```python
from build123d import *

# Parameters (mm, degrees)
SKETCH1_W                   = 57.3
SKETCH1_H                   = 42
BOSS_EXTRUDE1_DEPTH         = 6.35
TAP_DRILL_FOR_M3X0_5_TAP1_D = 3.25
CUT_EXTRUDE1_DEPTH          = 37.085246293
SKETCH5_W                   = 7.65
SKETCH5_H                   = 14.65
CUT_EXTRUDE2_DEPTH          = 37.085246293
FILLET1_R                   = 5


with BuildPart() as part:
    # Sketch1 → Boss-Extrude1 (new body)
    with BuildSketch(Plane.XY):
        Rectangle(SKETCH1_W, SKETCH1_H)
    extrude(amount=BOSS_EXTRUDE1_DEPTH)

    # Tap Drill for M3x0.5 Tap1 (through all)
    with Locations(Plane.XY.offset(6.35)):
        with Locations((15.5, 15.5), (15.5, -15.5), (-15.5, 15.5), (-15.5, -15.5)):
            Hole(TAP_DRILL_FOR_M3X0_5_TAP1_D / 2)

    # Sketch4 → Cut-Extrude1 (cut, through all)
    with BuildSketch(Plane.XY.offset(6.35)):
        with BuildLine():
            ThreePointArc((11, 0), (8.93028555, 6.422616289), (3.5, 10.428326807))
            Line((3.5, 10.428326807), (-3.5, 10.428326807))
            ThreePointArc((-3.5, 10.428326807), (-6.422616289, -8.93028555), (11, 0))
        make_face()
        with BuildLine():
            Line((-3.5, 10.428326807), (3.5, 10.428326807))
            ThreePointArc((3.5, 10.428326807), (0, 11), (-3.5, 10.428326807))
        make_face()
        with BuildLine():
            ThreePointArc((-3.5, 10.428326807), (0, 11), (3.5, 10.428326807))
            Line((3.5, 10.428326807), (3.5, 21))
            Line((3.5, 21), (-3.5, 21))
            Line((-3.5, 21), (-3.5, 10.428326807))
        make_face()
    extrude(amount=-CUT_EXTRUDE1_DEPTH, mode=Mode.SUBTRACT)

    # Sketch5 → Cut-Extrude2 (cut, through all)
    with BuildSketch(Plane.XY.offset(6.35)):
        with Locations((-24.825, 13.675)):
            Rectangle(SKETCH5_W, SKETCH5_H)
        with Locations((-24.825, -13.675)):
            Rectangle(SKETCH5_W, SKETCH5_H)
    cut_extrude2 = extrude(amount=-CUT_EXTRUDE2_DEPTH, mode=Mode.SUBTRACT)

    # Mirror1: Cut-Extrude2 across plane
    add(cut_extrude2.mirror(Plane(origin=(0, 0, 0), x_dir=(0, 0, 1), z_dir=(1, 0, 0))), mode=Mode.SUBTRACT)

    # Fillet1
    fillet1_edges = [part.edges().sort_by_distance(p)[0] for p in [
        (3.5, 10.428326807, 3.175),
        (-3.5, 10.428326807, 3.175),
        (-3.5, 21, 3.175),
        (3.5, 21, 3.175),
        (-21, 21, 3.175),
        (-21, -21, 3.175),
        (21, 21, 3.175),
        (21, -21, 3.175),
    ]]
    fillet(fillet1_edges, radius=FILLET1_R)


solid = part.part
```
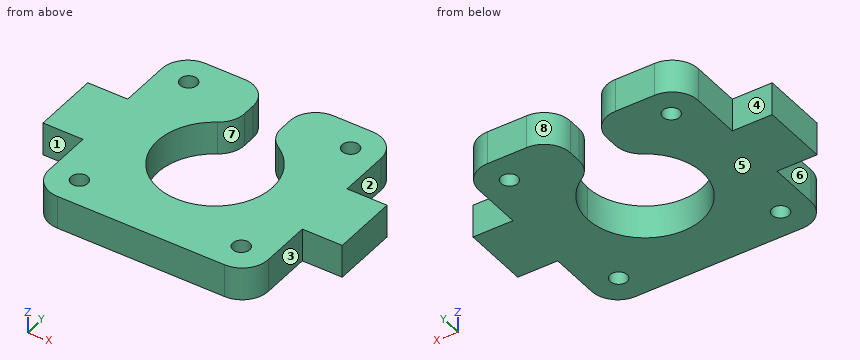
The model under review builds one solid part; all positions refer to its coordinate system, in mm. Face numbers are marked on the shaded views. A direction names the side the tool comes from. Round coordinates to 2 decimals unless told otherwise and drop trailing zeros. Write each loop counter-clockwise with the first axis right and the second up, starting at its lowest first coordinate (ties: lowest second). Pieces come first, ordered by that corner, then holes.
(1) Insertion check: pin 1 (2.5 mm diameter, centred on y = 15, z = 3, fed in from -X); pin 2 (1.9 mm diameter, centred on y = -10.5, z = 4.5, fed in from +X); pin 3 (2 mm diameter, centred on x = -19.5, y = 2, fed in from -Z); pin 4 (3 mm diameter, centred on x = -26.5, z = 1.5, fed in from +Y). Each pin has a flat end and moves straight along its axis. Give the tip position at first contact, or say it passes through.
(2) Machinability: for the marked faces 1, 2, 3 and 4, which of the approach directions +Z, -Z, +X, -X, +Y, -Y give a long, thin tool a straight path to every point of the face, cutting with its end or side? Answer none if there is none.
(3) We need section B-B on y = 10. Give the boundary of the cut face in (x, z).
(4) Wall thickness on L1, parallel to Y at x = 15.5, z = 1.5 (3 decimals); L2, parallel to X at y = -16, z = 1; L3, parallel to Y at x = -24.5, z = 5.75: over which ranges is each line inside the solid? List them lowest first.
(5) We need section D-D on x = 0. Give the boundary of the cut face in (y, z), and give its area (3 significant figures).
(6) Mouldability with a two-part tool opening along X and no side actions: class the marked faces 5, 6, 7 and 8 as +X half, -X half, draft (parallel to the pull), parting line (faces both ways), or undercut.
(7) We need section C-C on x = -7.5. Give the boundary of the cut face in (y, z), and give its area (3 significant figures).
(8) We need section A-A on z = 5.25. Give the boundary of the cut face in (x, y) (3 decimals).
Findings below:
1. pin 1: stops at x = -21
1. pin 2: stops at x = 21
1. pin 3: stops at z = 0
1. pin 4: stops at y = 6.35
2. face 1: +Z, -Z, -X, -Y
2. face 2: +Z, -Z, +X, +Y
2. face 3: +Z, -Z, +X, -Y
2. face 4: +Z, -Z, -X, +Y
3. outline: (-21, 0) - (-4.98, 0) - (-4.98, 6.35) - (-21, 6.35) - close; (4.98, 0) - (21, 0) - (21, 6.35) - (4.98, 6.35) - close
4. L1: y = -21 to -17.125, -13.875 to 13.875, 17.125 to 21
4. L2: x = -21 to -17.05, -13.95 to 13.95, 17.05 to 21
4. L3: y = -6.35 to 6.35
5. outline: (-21, 0) - (-11, 0) - (-11, 6.35) - (-21, 6.35) - close
5. area: 63.5 mm2
6. face 5: draft
6. face 6: -X half
6. face 7: undercut
6. face 8: undercut
7. outline: (-21, 0) - (-8.05, 0) - (-8.05, 6.35) - (-21, 6.35) - close; (8.05, 0) - (20.9, 0) - (20.9, 6.35) - (8.05, 6.35) - close
7. area: 164 mm2
8. outline: (-28.65, -6.35) - (-21, -6.35) - (-21, -16) arc R5 ccw to (-16, -21) - (16, -21) arc R5 ccw to (21, -16) - (21, -6.35) - (28.65, -6.35) - (28.65, 6.35) - (21, 6.35) - (21, 16) arc R5 ccw to (16, 21) - (8.5, 21) arc R5 ccw to (3.5, 16) - (3.5, 13.555) arc R5 ccw to (5.844, 9.319) arc R11 cw (long way) to (-5.844, 9.319) arc R5 ccw to (-3.5, 13.555) - (-3.5, 16) arc R5 ccw to (-8.5, 21) - (-16, 21) arc R5 ccw to (-21, 16) - (-21, 6.35) - (-28.65, 6.35) - close; hole circle Ø3.25 at (-15.5, -15.5); hole circle Ø3.25 at (-15.5, 15.5); hole circle Ø3.25 at (15.5, -15.5); hole circle Ø3.25 at (15.5, 15.5)
